```python
from build123d import *

# Parameters (mm, degrees)
BOSS_EXTRUDE1_DEPTH = 2
BOSS_EXTRUDE2_DEPTH = 0.25
SKETCH3_W           = 15.6
SKETCH3_H           = 10.74
CUT_EXTRUDE1_DEPTH  = 0.25
SKETCH4_R           = 7
BOSS_EXTRUDE3_DEPTH = 2
SKETCH5_R           = 6
BOSS_EXTRUDE4_DEPTH = 1.4
SKETCH6_R           = 2.85
BOSS_EXTRUDE5_DEPTH = 0.2
BOSS_EXTRUDE6_DEPTH = 3
SKETCH10_R          = 1
CUT_EXTRUDE4_DEPTH  = 3


with BuildPart() as part:
    # Sketch1 → Boss-Extrude1 (new body)
    with BuildSketch(Plane(origin=(0, 0, 0), x_dir=(1, 0, 0), z_dir=(0, 1, 0))):
        with BuildLine():
            ThreePointArc((5, 13.05), (0, 15.55), (-5, 13.05))
            Line((-5, 13.05), (-8, 13.05))
            ThreePointArc((-8, 13.05), (-8.70710678, 12.757106782), (-9, 12.050000002))
            Line((-9, 12.050000002), (-9, -6.591101056))
            ThreePointArc((-9, -6.591101056), (0, -20.95), (9, -6.591101056))
            Line((9, -6.591101056), (9, 12.05))
            ThreePointArc((9, 12.05), (8.707106781, 12.757106781), (8, 13.05))
            Line((8, 13.05), (5, 13.05))
        make_face()
    extrude(amount=BOSS_EXTRUDE1_DEPTH)

    # Sketch2 → Boss-Extrude2 (add)
    with BuildSketch(Plane(origin=(0, 2, 0), x_dir=(-1, 0, 0), z_dir=(0, 1, 0))):
        with BuildLine():
            Line((-8.000000002, -13.05), (8, -13.05))
            ThreePointArc((8, -13.05), (8.707106781, -12.757106781), (9, -12.05))
            Line((9, -12.05), (9, -0.41))
            ThreePointArc((9, -0.41), (8.853553391, -0.056446609), (8.5, 0.09))
            Line((8.5, 0.09), (-8.5, 0.09))
            ThreePointArc((-8.5, 0.09), (-8.853553391, -0.056446609), (-9, -0.41))
            Line((-9, -0.41), (-9, -12.05))
            ThreePointArc((-9, -12.05), (-8.707106782, -12.757106781), (-8.000000002, -13.05))
        make_face()
    extrude(amount=BOSS_EXTRUDE2_DEPTH)

    # Sketch3 → Cut-Extrude1 (cut)
    with BuildSketch(Plane(origin=(0, 2.25, 0), x_dir=(-1, 0, 0), z_dir=(0, 1, 0))):
        with Locations((0, -6.48)):
            Rectangle(SKETCH3_W, SKETCH3_H)
    extrude(amount=-CUT_EXTRUDE1_DEPTH, mode=Mode.SUBTRACT)

    # Sketch4 → Boss-Extrude3 (add)
    with BuildSketch(Plane(origin=(0, 2, 0), x_dir=(-1, 0, 0), z_dir=(0, 1, 0))):
        with Locations((0, 10.95)):
            Circle(SKETCH4_R)
    extrude(amount=BOSS_EXTRUDE3_DEPTH)

    # Sketch5 → Boss-Extrude4 (add)
    with BuildSketch(Plane(origin=(0, 4, 0), x_dir=(-1, 0, 0), z_dir=(0, 1, 0))):
        with Locations((0, 10.95)):
            Circle(SKETCH5_R)
    extrude(amount=BOSS_EXTRUDE4_DEPTH)

    # Sketch6 → Boss-Extrude5 (add)
    with BuildSketch(Plane(origin=(0, 5.4, 0), x_dir=(-1, 0, 0), z_dir=(0, 1, 0))):
        with Locations((0, 10.95)):
            Circle(SKETCH6_R)
    extrude(amount=BOSS_EXTRUDE5_DEPTH)

    # Sketch9 → Boss-Extrude6 (add)
    with BuildSketch(Plane(origin=(0, 5.6, 0), x_dir=(-1, 0, 0), z_dir=(0, 1, 0))):
        Polygon((-0.356289813, 8.243710187), (0, 8.6), (0.356289813, 8.243710187), (0.608224756, 8.680074308), (1.044588877, 8.428139365), (1.175, 8.914840301), (1.661700936, 8.784429178), (1.661700936, 9.288299064), (2.165570822, 9.288299064), (2.035159699, 9.775), (2.521860635, 9.905411123), (2.269925692, 10.341775244), (2.706289813, 10.593710187), (2.35, 10.95), (2.706289813, 11.306289813), (2.269925692, 11.558224756), (2.521860635, 11.994588877), (2.035159699, 12.125), (2.165570822, 12.611700936), (1.661700936, 12.611700936), (1.661700936, 13.115570822), (1.175, 12.985159699), (1.044588877, 13.471860635), (0.608224756, 13.219925692), (0.356289813, 13.656289813), (0, 13.3), (-0.356289813, 13.656289813), (-0.608224756, 13.219925692), (-1.044588877, 13.471860635), (-1.175, 12.985159699), (-1.661700936, 13.115570822), (-1.661700936, 12.611700936), (-2.165570822, 12.611700936), (-2.035159699, 12.125), (-2.521860635, 11.994588877), (-2.269925692, 11.558224756), (-2.706289813, 11.306289813), (-2.35, 10.95), (-2.706289813, 10.593710187), (-2.269925692, 10.341775244), (-2.521860635, 9.905411123), (-2.035159699, 9.775), (-2.165570822, 9.288299064), (-1.661700936, 9.288299064), (-1.661700936, 8.784429178), (-1.175, 8.914840301), (-1.044588877, 8.428139365), (-0.608224756, 8.680074308), align=None)
    extrude(amount=BOSS_EXTRUDE6_DEPTH)

    # Sketch10 → Cut-Extrude4 (cut)
    with BuildSketch(Plane(origin=(0, 8.6, 0), x_dir=(-1, 0, 0), z_dir=(0, 1, 0))):
        with Locations((0, 10.95)):
            Circle(SKETCH10_R)
    extrude(amount=-CUT_EXTRUDE4_DEPTH, mode=Mode.SUBTRACT)


solid = part.part
```
The listing builds one solid part. Answer for the finished solid, in the listing's coordinates (mm). A direction names the side the tool comes from. Round coordinates to 2 decimals unless told otherwise and drop trailing zeros. Loops run counter-clockwise (first coordinate to the right, second up) from the corner with the lowest first, then second, coordinate; pieces in that order, holes last.
1) Consider line 1 (Y direction, x = 1, z = 15.5); line 2 (Y direction, x = 1.25, z = -12); line 3 (Z direction, x = 1, y = 1). Determine where each line is inside the solid, lowest interval first.
Outcome:
line 1: y = 0 to 5.4
line 2: y = 0 to 2.25
line 3: z = -15.47 to 20.9
2) For a pull along Z with two mould halves and no side action, classify faces 5 (the face through (0, 5.6, 11)), 6 (the face through (-9, 1, -3)), 7 (the face through (4, 2, 5)), 8 (the face through (1.301, 4.69, 5.093)) as released by +Z, released by -Z, zero draft, split by the parting line, or undercut.
Outcome:
face 5: undercut
face 6: zero draft
face 7: undercut
face 8: split by the parting line
3) For faces 1 (the face through (9, 1, -3)), 2 (the face through (0, 2, -14)), 3 (the face through (1.517, 2.986, 4.116)), 4 (the face through (-5.2, 1.1, -13.05)), determine the directions among +Z, -Z, +X, -X, +Y, -Y from which every point of the face is accessible in a straight line to the end or side of a thin tool.
Outcome:
face 1: -Z, +X, +Y, -Y
face 2: -Z, +X, -X, +Y
face 3: +Y
face 4: -Z, +Y
4) A cutting plane is placed at A-A on z = 3.5. Determine the outline of the cut face in (x, y), plus the area to 3 significant figures.
Outcome:
outline: (-9, 0) - (9, 0) - (9, 2) - (-9, 2) - close
area: 36.0 mm2
5) Given P1, Ø2.5, axis at y = 1.5, z = -6.5, coming from the -X side; P2, Ø12, axis at x = -5.5, z = -10.5, coming from the +Y side; P3, Ø5, axis at x = 3.5, y = 3, coming from the +Z side, each flat-ended and moving along its own axis, determine where each tip first touches the part or whether it passes through.
Outcome:
P1: stops at x = -9
P2: stops at y = 2.25
P3: stops at z = 20.88
